Verification items for the finished model (mm, model axes). Face numbers are marked on the shaded views. Coordinates: 2 decimals unless noted, no trailing zeros. Order: outer loops, then holes, each group sorted by start corner. A loop starts at its lowest first (then second) coordinate and runs counter-clockwise, first axis right, second up.
Q1. Depth check by flat-ended pin: P1, Ø1.5, axis at y = 8, z = -27, coming from the +X side; P2, Ø3, axis at x = 0, z = 54, coming from the -Y side; P3, Ø6, axis at y = 9, z = 6, coming from the +X side; P4, Ø1.5, axis at x = -26, y = 6.5, coming from the -Z side. Enter the tip coordinate at first touch or a pass-through.
Q2. Cross-section at D-D, the plane x = -15. Record the boundary of the cut face in (y, z), and give its area (3 significant figures).
Q3. Cross-section at B-B, the plane x = 0. Record the boundary of the cut face in (y, z).
Q4. Cross-section at C-C, the plane z = 14.5. Record the boundary of the cut face in (x, y).
Q5. Thickness scan on line 1 (Z direction, x = -1, y = 9.75); line 2 (X direction, y = 2.25, z = 0). Record the ranges inside material, lowest first.
Q6. Draft check along X on the marked faces 1, 2 and 3. Enter one of: pulls with the +X half, pulls with the -X half, needs draft (parallel to the pull), parting line crosses it, or undercut.
Q7. Cross-section at A-A, the plane z = 0. Record the boundary of the cut face in (x, y).
from build123d import *

# Parameters (mm, degrees)
SKETCH1_R           = 57.5
SKETCH1_R_2         = 39.25
BOSS_EXTRUDE1_DEPTH = 8
SKETCH3_R           = 57.5
SKETCH3_R_2         = 35
BOSS_EXTRUDE2_DEPTH = 2
SKETCH2_R           = 2
CUT_EXTRUDE1_DEPTH  = 25


with BuildPart() as part:
    # Sketch1 → Boss-Extrude1 (new body)
    with BuildSketch(Plane(origin=(0, 0, 0), x_dir=(1, 0, 0), z_dir=(0, 1, 0))):
        with Locations(Location((0, 0, 0), (0, 0, 270))):
            Circle(SKETCH1_R)
        with Locations(Location((0, 0, 0), (0, 0, 270))):
            Circle(SKETCH1_R_2, mode=Mode.SUBTRACT)
    extrude(amount=BOSS_EXTRUDE1_DEPTH)

    # Sketch3 → Boss-Extrude2 (add)
    with BuildSketch(Plane(origin=(0, 8, 0), x_dir=(1, 0, 0), z_dir=(0, 1, 0))):
        with Locations(Location((0, 0, 0), (0, 0, 270))):
            Circle(SKETCH3_R)
        with Locations(Location((0, 0, 0), (0, 0, 270))):
            Circle(SKETCH3_R_2, mode=Mode.SUBTRACT)
    extrude(amount=BOSS_EXTRUDE2_DEPTH)

    # Sketch2 → Cut-Extrude1 (cut)
    with BuildSketch(Plane(origin=(0, 10, 0), x_dir=(1, 0, 0), z_dir=(0, 1, 0))):
        with Locations(Location((0, 54, 0), (0, 0, 270))):
            Circle(SKETCH2_R)
        with Locations(Location((20.664905348, 49.889494756, 0), (0, 0, 270))):
            Circle(SKETCH2_R)
        with Locations(Location((38.183766184, 38.183766184, 0), (0, 0, 270))):
            Circle(SKETCH2_R)
        with Locations(Location((49.889494756, 20.664905348, 0), (0, 0, 270))):
            Circle(SKETCH2_R)
        with Locations(Location((54, 0, 0), (0, 0, 270))):
            Circle(SKETCH2_R)
        with Locations(Location((49.889494756, -20.664905348, 0), (0, 0, 270))):
            Circle(SKETCH2_R)
        with Locations(Location((38.183766184, -38.183766184, 0), (0, 0, 270))):
            Circle(SKETCH2_R)
        with Locations(Location((20.664905348, -49.889494756, 0), (0, 0, 270))):
            Circle(SKETCH2_R)
        with Locations(Location((0, -54, 0), (0, 0, 270))):
            Circle(SKETCH2_R)
        with Locations(Location((-20.664905348, -49.889494756, 0), (0, 0, 270))):
            Circle(SKETCH2_R)
        with Locations(Location((-38.183766184, -38.183766184, 0), (0, 0, 270))):
            Circle(SKETCH2_R)
        with Locations(Location((-49.889494756, -20.664905348, 0), (0, 0, 270))):
            Circle(SKETCH2_R)
        with Locations(Location((-54, 0, 0), (0, 0, 270))):
            Circle(SKETCH2_R)
        with Locations(Location((-49.889494756, 20.664905348, 0), (0, 0, 270))):
            Circle(SKETCH2_R)
        with Locations(Location((-38.183766184, 38.183766184, 0), (0, 0, 270))):
            Circle(SKETCH2_R)
        with Locations(Location((-20.664905348, 49.889494756, 0), (0, 0, 270))):
            Circle(SKETCH2_R)
    extrude(amount=-CUT_EXTRUDE1_DEPTH, mode=Mode.SUBTRACT)


solid = part.part
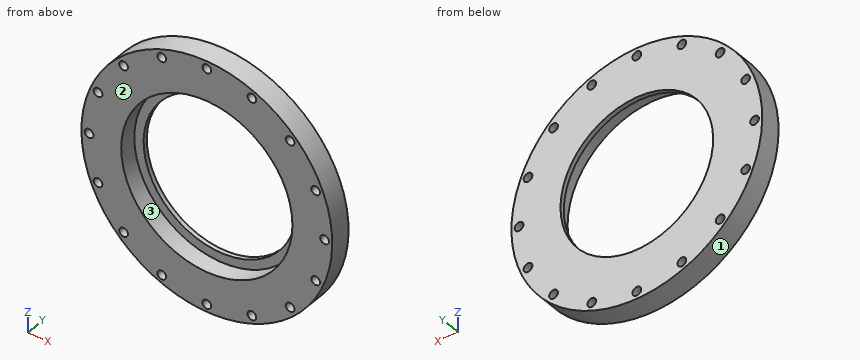
Check values:
1. P1: stops at x = 51.16
1. P2: passes through
1. P3: stops at x = 57.42
1. P4: stops at z = -51.66
2. outline: (0, -55.51) - (10, -55.51) - (10, -31.62) - (8, -31.62) - (8, -36.27) - (0, -36.27) - close; (0, 36.27) - (8, 36.27) - (8, 31.62) - (10, 31.62) - (10, 55.51) - (0, 55.51) - close
2. area: 403 mm2
3. outline: (0, -57.5) - (10, -57.5) - (10, -56) - (0, -56) - close; (0, -52) - (10, -52) - (10, -35) - (8, -35) - (8, -39.25) - (0, -39.25) - close; (0, 39.25) - (8, 39.25) - (8, 35) - (10, 35) - (10, 52) - (0, 52) - close; (0, 56) - (10, 56) - (10, 57.5) - (0, 57.5) - close
4. outline: (-55.64, 0) - (-36.47, 0) - (-36.47, 8) - (-31.86, 8) - (-31.86, 10) - (-55.64, 10) - close; (31.86, 8) - (36.47, 8) - (36.47, 0) - (55.64, 0) - (55.64, 10) - (31.86, 10) - close
5. line 1: z = -57.49 to -55.73, -52.27 to -34.99, 34.99 to 52.27, 55.73 to 57.49
5. line 2: x = -57.5 to -56, -52 to -39.25, 39.25 to 52, 56 to 57.5
6. face 1: parting line crosses it
6. face 2: needs draft
6. face 3: undercut
7. outline: (-57.5, 0) - (-56, 0) - (-56, 10) - (-57.5, 10) - close; (-52, 0) - (-39.25, 0) - (-39.25, 8) - (-35, 8) - (-35, 10) - (-52, 10) - close; (35, 8) - (39.25, 8) - (39.25, 0) - (52, 0) - (52, 10) - (35, 10) - close; (56, 0) - (57.5, 0) - (57.5, 10) - (56, 10) - close
